```python
from build123d import *

# Parameters (mm, degrees)
SKETCH1_R           = 5.1
SKETCH1_R_2         = 1.25
BOSS_EXTRUDE1_DEPTH = 3
FILLET1_R           = 1.5
SKETCH3_R           = 1.5
CUT_EXTRUDE2_DEPTH  = 3
SKETCH4_W           = 33.045580095
SKETCH4_H           = 44
CUT_EXTRUDE3_DEPTH  = 10
FILLET2_R           = 5


with BuildPart() as part:
    # Sketch1 → Boss-Extrude1 (new body)
    with BuildSketch(Plane(origin=(0, 0, 0), x_dir=(1, 0, 0), z_dir=(0, 1, 0))):
        with BuildLine():
            Line((128, 22), (0, 22))
            Line((0, 22), (0, 16.492422502))
            ThreePointArc((0, 16.492422502), (8, 0), (0, -16.492422502))
            Line((0, -16.492422502), (0, -22))
            Line((0, -22), (128, -22))
            ThreePointArc((128, -22), (150, 0), (128, 22))
        make_face()
        with Locations(Location((128, 0, 0), (0, 0, 270))):
            Circle(SKETCH1_R, mode=Mode.SUBTRACT)
        with Locations(Location((117.837325142, 4.209517756, 0), (0, 0, 270))):
            Circle(SKETCH1_R_2, mode=Mode.SUBTRACT)
        with Locations(Location((123.790482244, 10.162674858, 0), (0, 0, 270))):
            Circle(SKETCH1_R_2, mode=Mode.SUBTRACT)
        with Locations(Location((132.209517756, 10.162674858, 0), (0, 0, 270))):
            Circle(SKETCH1_R_2, mode=Mode.SUBTRACT)
        with Locations(Location((138.162674858, 4.209517756, 0), (0, 0, 270))):
            Circle(SKETCH1_R_2, mode=Mode.SUBTRACT)
        with Locations(Location((138.162674858, -4.209517756, 0), (0, 0, 270))):
            Circle(SKETCH1_R_2, mode=Mode.SUBTRACT)
        with Locations(Location((132.209517756, -10.162674858, 0), (0, 0, 270))):
            Circle(SKETCH1_R_2, mode=Mode.SUBTRACT)
        with Locations(Location((5, 17.3, 0), (0, 0, 270))):
            Circle(SKETCH1_R_2, mode=Mode.SUBTRACT)
        with Locations(Location((27, 17.3, 0), (0, 0, 270))):
            Circle(SKETCH1_R_2, mode=Mode.SUBTRACT)
        with Locations(Location((27, -17.3, 0), (0, 0, 90))):
            Circle(SKETCH1_R_2, mode=Mode.SUBTRACT)
        with Locations(Location((5, -17.3, 0), (0, 0, 90))):
            Circle(SKETCH1_R_2, mode=Mode.SUBTRACT)
        with Locations(Location((123.790482244, -10.162674858, 0), (0, 0, 270))):
            Circle(SKETCH1_R_2, mode=Mode.SUBTRACT)
        with Locations(Location((117.837325142, -4.209517756, 0), (0, 0, 270))):
            Circle(SKETCH1_R_2, mode=Mode.SUBTRACT)
        with Locations(Location((34.8, 11, 0), (0, 0, 270))):
            Circle(SKETCH1_R_2, mode=Mode.SUBTRACT)
        with Locations(Location((34.8, -11, 0), (0, 0, 90))):
            Circle(SKETCH1_R_2, mode=Mode.SUBTRACT)
    extrude(amount=BOSS_EXTRUDE1_DEPTH)

    # Fillet1
    fillet1_edges = [part.edges().sort_by_distance(p)[0] for p in [
        (0, 1.5, 16.492422502),
        (0, 1.5, -16.492422502),
        (0, 1.5, -22),
        (0, 1.5, 22),
    ]]
    fillet(fillet1_edges, radius=FILLET1_R)

    # Sketch3 → Cut-Extrude2 (cut)
    with BuildSketch(Plane(origin=(0, 3, 0), x_dir=(1, 0, 0), z_dir=(0, 1, 0))):
        with Locations(Location((45, 15, 0), (0, 0, 270))):
            Circle(SKETCH3_R)
        with Locations(Location((65, 15, 0), (0, 0, 270))):
            Circle(SKETCH3_R)
        with Locations(Location((85, 15, 0), (0, 0, 270))):
            Circle(SKETCH3_R)
        with Locations(Location((85, -15, 0), (0, 0, 90))):
            Circle(SKETCH3_R)
        with Locations(Location((65, -15, 0), (0, 0, 90))):
            Circle(SKETCH3_R)
        with Locations(Location((45, -15, 0), (0, 0, 90))):
            Circle(SKETCH3_R)
    extrude(amount=-CUT_EXTRUDE2_DEPTH, mode=Mode.SUBTRACT)

    # Sketch4 → Cut-Extrude3 (cut)
    with BuildSketch(Plane.XZ):
        with Locations((6.477209952, 0)):
            Rectangle(SKETCH4_W, SKETCH4_H)
    extrude(amount=-CUT_EXTRUDE3_DEPTH, mode=Mode.SUBTRACT)

    # Fillet2
    fillet2_edges = [part.edges().sort_by_distance(p)[0] for p in [
        (23, 1.5, 22),
        (23, 1.5, -22),
    ]]
    fillet(fillet2_edges, radius=FILLET2_R)


solid = part.part
```
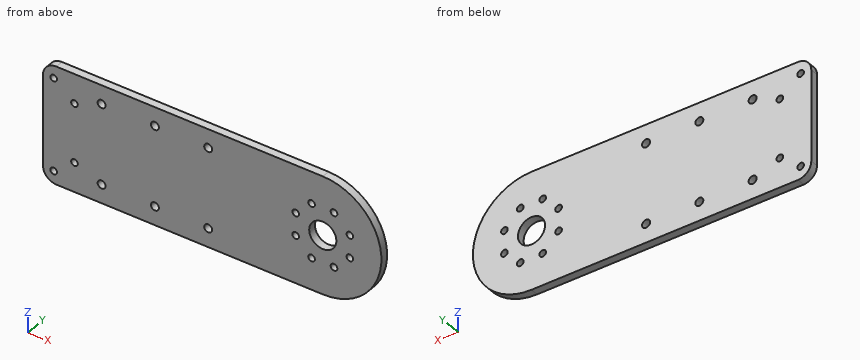
Can you work these out from the model? Positions are in its coordinate system, mm. Coordinates: 2 decimals unless noted, no trailing zeros. Write each loop counter-clockwise with the first axis right and the second up, starting at its lowest first coordinate (ties: lowest second). Pieces come first, ordered by that corner, then holes. Notation, with made-up numbers: M 1,70.5 L 32,70.5 A30 cw 32,93.5 Z; hole C -1,-22.75 d3. An arc over 180 degrees is marked long. Answer as CSV lines item,"result".
Item 1: I'm going to push a flat-ended pin straight in: P1, Ø2.5, axis at x = 65, z = 15, coming from the +Y side. Where does the tip first touch, or does it pass through?
Geometry results:
P1,"passes through"
Item 2: Imagine slicing it at C-C on y = 2.15. State how many separate pieces and enclosed holes the cut face has, plus the area to 3 significant figures.
Geometry results:
separate pieces,"1"
enclosed holes,"19"
area,"5,190 mm2"
Item 3: Imagine slicing it at A-A on z = 0. List the corners of the cut face in (x, y) for me.
Geometry results:
outline,"M 23,0 L 122.9,0 L 122.9,3 L 23,3 Z; M 133.1,0 L 150,0 L 150,3 L 133.1,3 Z"
Item 4: Imagine slicing it at B-B on x = 65. List the corners of the cut face in (y, z) for me, plus the area to 3 significant figures.
Geometry results:
outline,"M 0,-22 L 3,-22 L 3,-16.5 L 0,-16.5 Z; M 0,-13.5 L 3,-13.5 L 3,13.5 L 0,13.5 Z; M 0,16.5 L 3,16.5 L 3,22 L 0,22 Z"
area,"114 mm2"
Item 5: Please list where these lines run through material, in increasing order: line 1 along Z through (x, y) = (85, 1.35); line 2 along X through (y, z) = (1.4, -10); line 3 along Z through (x, y) = (123.5, 2.1).
Geometry results:
line 1,"z = -22 to -16.5, -13.5 to 13.5, 16.5 to 22"
line 2,"x = 23 to 34.05, 35.55 to 122.55, 125.03 to 130.97, 133.45 to 147.6"
line 3,"z = -22 to -11.38, -8.95 to -2.4, 2.4 to 8.95, 11.38 to 22"
